Verification items for the finished model (mm, model axes). Face numbers are marked on the shaded views. Coordinates: 2 decimals unless noted, no trailing zeros. Order: outer loops, then holes, each group sorted by start corner. A loop starts at its lowest first (then second) coordinate and runs counter-clockwise, first axis right, second up. Notation, with made-up numbers: M 41,89.5 L 51,89.5 A23 ccw 51,116.5 Z; hole C 9,38 d8. An arc over 180 degrees is marked long. Return JSON: item names as keys, results as strings. Group by question number.
1. Material ranges on line 1 along Y through (x, z) = (-0.75, -11.5); line 2 along Y through (x, z) = (-2, -2.5); line 3 along Y through (x, z) = (3.5, 2), recorded low to high.
2. Gauge pin test, flat ends, axial feed: pin 1 (2 mm diameter, centred on x = 3, z = 6, fed in from +Y); pin 2 (8 mm diameter, centred on y = 26, z = 0.5, fed in from -X); pin 3 (3 mm diameter, centred on y = 28.5, z = 4.5, fed in from +X). Record the tip position at first contact, or that the pin passes through.
3. Mould release check, pull along Y, two halves, no side actions. Record for the marked faces 1, 2, 3 and 4: +Y half, -Y half, draft (parallel to the pull), parting line (faces both ways), or undercut.
4. Section check A-A, the plane z = 11.25. Record the cut outline in (x, y).
```python
from build123d import *

# Parameters (mm, degrees)
SKETCH1_W           = 25.4
SKETCH1_H           = 25.4
BOSS_EXTRUDE1_DEPTH = 12.7
SKETCH2_R           = 2.54
REVOLVE1_ANGLE      = 180
BOSS_EXTRUDE2_REACH = 38.478
SKETCH2_3_R         = 2.54


with BuildPart() as part:
    # Sketch1 → Boss-Extrude1 (new, symmetric)
    with BuildSketch(Plane(origin=(0, 0, 0), x_dir=(1, 0, 0), z_dir=(0, 1, 0))):
        Rectangle(SKETCH1_W, SKETCH1_H)
    extrude(amount=BOSS_EXTRUDE1_DEPTH, both=True)

    # Sketch2_3 → Boss-Extrude2 (add, up to next)
    with BuildSketch(Plane(origin=(0, 19.05, 0), x_dir=(1, 0, 0), z_dir=(0, 1, 0)), mode=Mode.PRIVATE) as boss_extrude2_sk1:
        with Locations(Location((8.141095825, -8.141095825, 0), (0, 0, 315))):
            Circle(SKETCH2_3_R)
    boss_extrude2_tool1 = extrude(boss_extrude2_sk1.sketch, amount=-BOSS_EXTRUDE2_REACH, mode=Mode.PRIVATE) - part.part
    # Sketch2_3 → Boss-Extrude2 (add, up to next)
    with BuildSketch(Plane(origin=(0, 19.05, 0), x_dir=(1, 0, 0), z_dir=(0, 1, 0)), mode=Mode.PRIVATE) as boss_extrude2_sk2:
        with Locations(Location((-8.141095825, 8.141095825, 0), (0, 0, 135))):
            Circle(SKETCH2_3_R)
    boss_extrude2_tool2 = extrude(boss_extrude2_sk2.sketch, amount=-BOSS_EXTRUDE2_REACH, mode=Mode.PRIVATE) - part.part


with BuildPart() as body_2:
    # Sketch2 → Revolve1 (revolve)
    with BuildSketch(Plane(origin=(0, 19.05, 0), x_dir=(1, 0, 0), z_dir=(0, 1, 0))):
        with Locations((8.141095825, -8.141095825)):
            Circle(SKETCH2_R)
    revolve(axis=Axis((0, 19.05, 0), (-0.7071067811865464, 0, 0.7071067811865487)), revolution_arc=REVOLVE1_ANGLE)


with BuildPart() as part_1:
    add(part.part)

    add(body_2.part)  # Boss-Extrude2 merges body 2
    add(boss_extrude2_tool1.solids().sort_by_distance((8.141096, 19.05, 8.141096))[0])
    add(boss_extrude2_tool2.solids().sort_by_distance((-8.141096, 19.05, -8.141096))[0])


solid = part_1.part
```
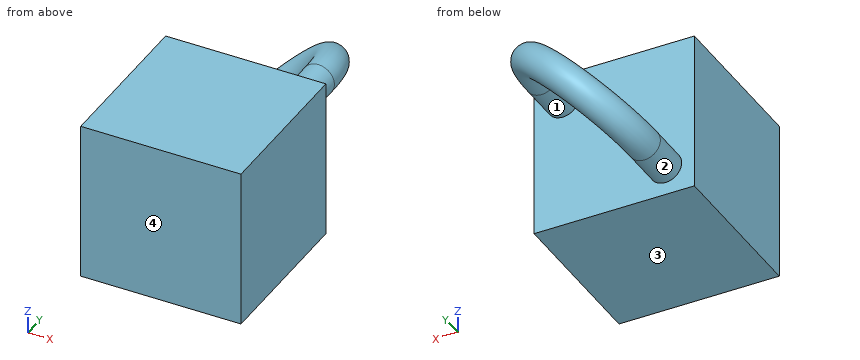
Answers follow:
{
 "1": {"line 1": "-12.7 to 12.7", "line 2": "-12.7 to 12.7, 27.47 to 32.71", "line 3": "-12.7 to 12.7, 27.39 to 32.31"},
 "2": {"pin 1": "y = 31.46", "pin 2": "x = -6.78", "pin 3": "x = 8.48"},
 "3": {"face 1": "undercut", "face 2": "undercut", "face 3": "draft", "face 4": "-Y half"},
 "4": {"outline": "M -12.7,-12.7 L 12.7,-12.7 L 12.7,12.7 L -12.7,12.7 Z"}
}
